Geometry check sheet. Reference: the model listing, model coordinates, mm. Face numbers are marked on the shaded views. A direction names the side the tool comes from. Coordinates: 2 decimals unless noted, no trailing zeros. Loops run counter-clockwise (first coordinate to the right, second up) from the corner with the lowest first, then second, coordinate; pieces in that order, holes last. Notation, with made-up numbers: M 84,80 L 94,80 A23 ccw 94,107 Z; hole C 50,55.5 d9. An arc over 180 degrees is marked long. Use CSV: the item, a comma, the result in double quotes.
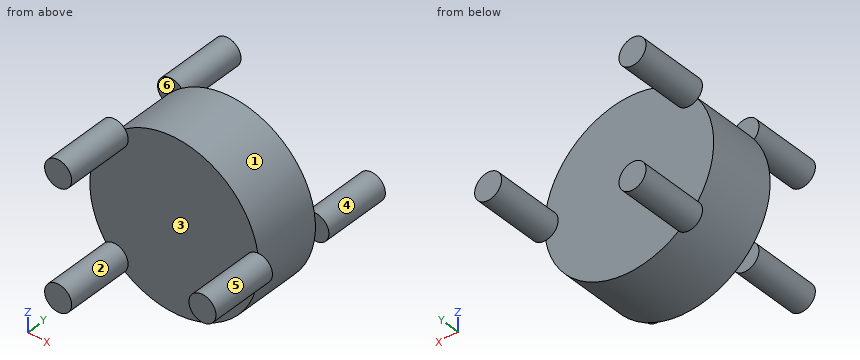
```python
from build123d import *

# Parameters (mm, degrees)
SKETCH7_R           = 12.5
BOSS_EXTRUDE2_DEPTH = 10
SKETCH8_R           = 2
BOSS_EXTRUDE3_DEPTH = 10
SKETCH9_R           = 2
BOSS_EXTRUDE4_DEPTH = 10
BOSS_EXTRUDE5_START = 10
SKETCH12_R          = 2
BOSS_EXTRUDE5_DEPTH = 10
BOSS_EXTRUDE6_START = 10
SKETCH13_R          = 2
BOSS_EXTRUDE6_DEPTH = 10


with BuildPart() as part:
    # Sketch7 → Boss-Extrude2 (new body)
    with BuildSketch(Plane(origin=(0, 0, 0), x_dir=(1, 0, 0), z_dir=(0, 1, 0))):
        with Locations(Location((0, 0, 0), (0, 0, 270))):
            Circle(SKETCH7_R)
    extrude(amount=BOSS_EXTRUDE2_DEPTH)

    # Sketch8 → Boss-Extrude3 (add)
    with BuildSketch(Plane(origin=(0, 10, 0), x_dir=(1, 0, 0), z_dir=(0, 1, 0))):
        with Locations(Location((-8.838834765, 8.838834765, 0), (0, 0, 40.411434264))):
            Circle(SKETCH8_R)
    boss_extrude3 = extrude(amount=BOSS_EXTRUDE3_DEPTH)

    # Mirror1: Boss-Extrude3 across plane
    add(boss_extrude3.mirror(Plane.XY))

    # Sketch9 → Boss-Extrude4 (add)
    with BuildSketch(Plane(origin=(0, 10, 0), x_dir=(1, 0, 0), z_dir=(0, 1, 0))):
        with Locations(Location((12.5, 0, 0), (0, 0, 94.588565736))):
            Circle(SKETCH9_R)
    extrude(amount=BOSS_EXTRUDE4_DEPTH)

    # Sketch12 → Boss-Extrude5 (add)
    with BuildSketch(Plane.XZ.offset(BOSS_EXTRUDE5_START)):
        with Locations(Location((-8.838834765, -8.838834765, 0), (0, 0, 319.588565736))):
            Circle(SKETCH12_R)
    boss_extrude5 = extrude(amount=-BOSS_EXTRUDE5_DEPTH)

    # Mirror3: Boss-Extrude5 across plane
    add(boss_extrude5.mirror(Plane.XY))

    # Sketch13 → Boss-Extrude6 (add)
    with BuildSketch(Plane(origin=(0, 0, 0), x_dir=(-1, 0, 0), z_dir=(0, -1, 0)).offset(BOSS_EXTRUDE6_START)):
        with Locations(Location((-12.5, 0, 0), (0, 0, 85.411434264))):
            Circle(SKETCH13_R)
    extrude(amount=-BOSS_EXTRUDE6_DEPTH)


solid = part.part
```
1. Thickness scan on line 1 (Y direction, x = -8.5, z = 10.25); line 2 (Y direction, x = -5.5, z = -5); line 3 (X direction, y = -2.75, z = 10.5). Record the ranges inside material, lowest first. Write a range as [from, to].
The answers:
line 1,"[-10, 0], [10, 20]"
line 2,"[0, 10]"
line 3,"[-9.95, -7.73]"
2. Section check B-B, the plane x = 0. Record the cut outline in (y, z), plus the area to 3 significant figures.
The answers:
outline,"M 0,-12.5 L 10,-12.5 L 10,12.5 L 0,12.5 Z"
area,"250 mm^2"
3. Gauge pin test, flat ends, axial feed: P1, Ø2, axis at y = 13, z = 6.5, coming from the +X side; P2, Ø1, axis at x = 2.5, y = 8, coming from the +Z side; P3, Ø1.5, axis at x = -9.5, z = 6, coming from the -Y side; P4, Ø10, axis at x = 3.5, y = 10.5, coming from the +Z side. Record the tip position at first contact, or that the pin passes through.
The answers:
P1,"x = -7.35"
P2,"z = 12.34"
P3,"y = 0"
P4,"z = 12.5"
4. Section check A-A, the plane z = -9.5. Record the cut outline in (x, y), plus the area to 3 significant figures.
The answers:
outline,"M -10.73,-10 L -6.95,-10 L -6.95,0 L 8.12,0 L 8.12,10 L -6.95,10 L -6.95,20 L -10.73,20 L -10.73,10 L -8.12,10 L -8.12,0 L -10.73,0 Z"
area,"238 mm^2"
5. Set-up check for the marked faces 4, 5 and 6: record each of +Z, -Z, +X, -X, +Y, -Y from which the full face is reachable in a straight line by a thin tool's end or side.
The answers:
face 4,"+Y"
face 5,"-Y"
face 6,"+Z, -X"
6. Release check for a two-part mould opening along Y. For the marked faces 1, 2 and 3 record: +Y half, -Y half, draft (parallel to the pull), parting line (faces both ways), or undercut.
The answers:
face 1,"undercut"
face 2,"draft"
face 3,"-Y half"
7. Section check D-D, the plane z = 0. Record the cut outline in (x, y), plus the area to 3 significant figures.
The answers:
outline,"M -12.5,0 L 10.5,0 L 10.5,-10 L 14.5,-10 L 14.5,0 L 12.5,0 L 12.5,10 L 14.5,10 L 14.5,20 L 10.5,20 L 10.5,10 L -12.5,10 Z"
area,"330 mm^2"
8. Section check C-C, the plane y = 8.25. Record the cut outline in (x, z), plus the area to 3 significant figures.
The answers:
outline,"C 0,0 d25"
area,"491 mm^2"
